Here's how the part is built. I have some questions about the finished solid (model axes, mm). Face numbers are marked on the shaded views. Coordinates: 2 decimals unless noted, no trailing zeros. Write each loop counter-clockwise with the first axis right and the second up, starting at its lowest first coordinate (ties: lowest second). Pieces come first, ordered by that corner, then holes. Notation, with made-up numbers: (0, 61.25) - (28, 61.25) arc R26 cw to (28, 94.25) - close; hole circle Ø6 at (-26.75, 37). An arc over 180 degrees is marked (long way). Answer in a Markdown table with one row per item. Add a question column.
Item 1: We'd pull the mould along X, two halves only. Please class the marked faces 1, 2 and 3: +X half, -X half, draft (parallel to the pull), parting line (faces both ways), or undercut.
Item 2: If I drill on probe 1 along X at (y, z) = (-0.5, -12.5); probe 2 along X at (y, z) = (0, -22); probe 3 along Z at (x, y) = (320, 1.5), over which ranges is the centre line in solid material (lowest first)? Write a range as from..to.
Item 3: Imagine slicing it at B-B (x = 7). Please give me the cut outline in (y, z) (3 decimals).
Item 4: Imagine slicing it at A-A (y = 0). Please give me the cut outline in (x, z) (3 decimals), plus the area to 3 significant figures.
Item 5: Imagine slicing it at C-C (x = 233). Please give me the cut outline in (y, z).
Item 6: I'm going to push flat-ended pins straight in: pin 1 (5 mm diameter, centred on x = -7, z = 1, fed in from +Y); pin 2 (12 mm diameter, centred on y = -7, z = -20.5, fed in from +X); pin 3 (1 mm diameter, centred on x = 177, z = 0, fed in from -Y); pin 4 (14 mm diameter, centred on x = -27.5, z = -13.5, fed in from -Y). Where does each tip first touch, or does it pass through?
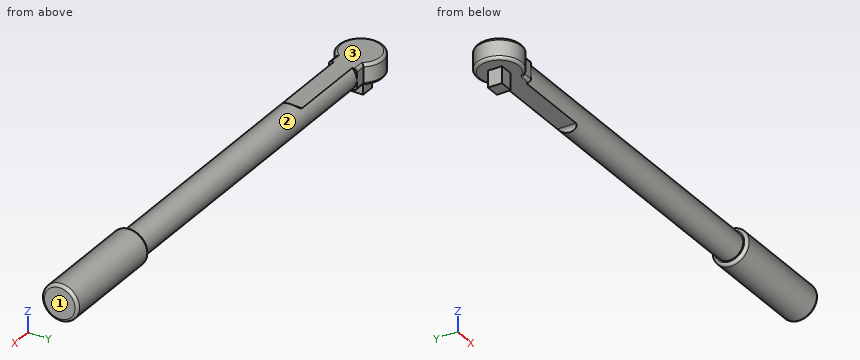
from build123d import *

# Parameters (mm, degrees)
F0_R        = 12.7
F1_DEPTH    = 406.4
F2_R        = 16.51
F3_DEPTH    = 101.6
F5_DEPTH    = 9.525
F6_W        = 76.2
F6_H        = 3.175
F7_DEPTH    = 12.7
F8_T4_DEPTH = 42.2005208253
F8_S5_R     = 12.7
F8_T6_DEPTH = 23
F9_T4_DEPTH = 42.2005208253
F9_S5_R     = 12.7
F9_T6_DEPTH = 23
F10_R       = 2.54
F11_W       = 12.7
F11_H       = 12.7
F12_DEPTH   = 15.24


# Not quite as in the source:
# - a fillet or chamfer that OpenCascade refuses, or shapes differently, is made with other operations: its cross-section is extruded or revolved along the edge and cut away or added


with BuildPart() as f1:
    # F0 (on Right) → F1 (new body)
    with BuildSketch(Plane.YZ):
        Circle(F0_R)
    extrude(amount=F1_DEPTH)

    # F2 (on face) → F3 (join)
    with BuildSketch(Plane.YZ.offset(406.4)):
        Circle(F2_R)
    extrude(amount=-F3_DEPTH)

    # F4 (on Top) → F5 (join, symmetric)
    with BuildSketch(Plane.XY):
        with BuildLine():
            Line((0, 12.7), (-9.5377050841, 12.7))
            ThreePointArc((-9.5377050841, 12.7), (-45.72, 0), (-9.5377050841, -12.7))
            Line((-9.5377050841, -12.7), (0, -12.7))
            Line((0, -12.7), (0, 12.7))
        make_face()
    extrude(amount=F5_DEPTH, both=True)

    # F6 (on Front) → F7 (cut, symmetric)
    with BuildSketch(Plane.XZ):
        with Locations((38.1, 11.1125)):
            Rectangle(F6_W, F6_H)
        with Locations((38.1, -11.1125)):
            Rectangle(F6_W, F6_H)
    extrude(amount=F7_DEPTH, both=True, mode=Mode.SUBTRACT)

    # F8: fillet of radius 5.08 on 1 edges, made by hand


with BuildPart() as f8_tool2:
    # F8_s3 → F8_t4 (new body)
    with BuildSketch(Plane.XZ.offset(-21.1002604126)):
        with BuildLine():
            ThreePointArc((76.2, 14.605), (74.7121024484, 11.0128975516), (71.12, 9.525))
            Line((71.12, 9.525), (76.2, 9.525))
            Line((76.2, 9.525), (76.2, 14.605))
        make_face()
    extrude(amount=F8_T4_DEPTH)

    # F8_s5 → F8_t6 (intersect, symmetric)
    with BuildSketch(Plane.YZ.offset(73.7)):
        Circle(F8_S5_R)
    extrude(amount=F8_T6_DEPTH, both=True, mode=Mode.INTERSECT)


with BuildPart() as f1_1:
    add(f1.part)

    # F8_t1: union F8_tool2
    add(f8_tool2.part)

    # F9: fillet of radius 5.08 on 1 edges, made by hand


with BuildPart() as f9_tool2:
    # F9_s3 → F9_t4 (new body)
    with BuildSketch(Plane.XZ.offset(21.1002604126)):
        with BuildLine():
            ThreePointArc((71.12, -9.525), (74.7121024484, -11.0128975516), (76.2, -14.605))
            Line((76.2, -14.605), (76.2, -9.525))
            Line((76.2, -9.525), (71.12, -9.525))
        make_face()
    extrude(amount=-F9_T4_DEPTH)

    # F9_s5 → F9_t6 (intersect, symmetric)
    with BuildSketch(Plane.YZ.offset(73.7)):
        Circle(F9_S5_R)
    extrude(amount=F9_T6_DEPTH, both=True, mode=Mode.INTERSECT)


with BuildPart() as f1_2:
    add(f1_1.part)

    # F9_t1: union F9_tool2
    add(f9_tool2.part)

    # F10
    f10_edges = [f1_2.edges().sort_by_distance(p)[0] for p in [
        (-45.72, 0, -9.525),
        (-45.72, 0, 9.525),
        (-4.768853, -12.7, -9.525),
        (-4.768853, -12.7, 9.525),
        (-4.768853, 12.7, -9.525),
        (-4.768853, 12.7, 9.525),
        (406.4, -16.51, 0),
        (304.8, -16.51, 0),
    ]]
    fillet(f10_edges, radius=F10_R)

    # F11 (on face) → F12 (join)
    with BuildSketch(Plane(origin=(0, 0, -9.525), x_dir=(1, 0, 0), z_dir=(0, 0, -1))):
        with Locations((-25.4, 0)):
            Rectangle(F11_W, F11_H)
    extrude(amount=F12_DEPTH)


solid = f1_2.part
Here are the results:
| question | item | result |
|---|---|---|
| 1 | face 1 | +X half |
| 1 | face 2 | undercut |
| 1 | face 3 | draft |
| 2 | probe 1 | x = -31.75..-19.05, 75.74..406.4 |
| 2 | probe 2 | x = -31.75..-19.05 |
| 2 | probe 3 | z = -16.44..16.44 |
| 3 | outline | (-8.4, -9.525) - (8.4, -9.525) arc R12.7 ccw to (8.4, 9.525) - (-8.4, 9.525) arc R12.7 ccw to start |
| 4 | outline | (-45.72, -6.985) arc R2.54 ccw to (-43.18, -9.525) - (-31.75, -9.525) - (-31.75, -24.765) - (-19.05, -24.765) - (-19.05, -9.525) - (71.12, -9.525) arc R5.08 cw to (75.829, -12.7) - (304.8, -12.7) - (304.8, -13.97) arc R2.54 ccw to (307.34, -16.51) - (403.86, -16.51) arc R2.54 ccw to (406.4, -13.97) - (406.4, 13.97) arc R2.54 ccw to (403.86, 16.51) - (307.34, 16.51) arc R2.54 ccw to (304.8, 13.97) - (304.8, 12.7) - (75.829, 12.7) arc R5.08 cw to (71.12, 9.525) - (-43.18, 9.525) arc R2.54 ccw to (-45.72, 6.985) - close |
| 4 | area | 11,700 mm2 |
| 5 | outline | circle Ø25.4 at (0, 0) |
| 6 | pin 1 | stops at y = 12.7 |
| 6 | pin 2 | stops at x = 405.75 |
| 6 | pin 3 | stops at y = -12.7 |
| 6 | pin 4 | stops at y = -20.32 |
